Work out the finished part from the listing and answer in its coordinate system (mm). A direction names the side the tool comes from. Coordinates: 2 decimals unless noted, no trailing zeros. Write each loop counter-clockwise with the first axis right and the second up, starting at its lowest first coordinate (ties: lowest second). Pieces come first, ordered by that corner, then holes. Notation, with made-up numbers: (25.5, 84.5) -> (79.5, 84.5) arc R19 ccw to (79.5, 104.5) -> close; hole circle Ø3 at (2.25, 72.25). An arc over 180 degrees is marked (long way). Write each question's results on one line, items separated by ' | '. Start each with the question number.
Autodesk Inventor part; units mm, degrees
ref_plane "Work Plane1" through (-11.4, -3, 12.9) normal (0, 0, -1) x (-1, 0, 0)
ref_plane "Work Plane3" through (-9.3294, -8.5807, 12.9) normal (-0.9659258, 0.258819, 0) x (-0.258819, -0.9659258, 0)
ref_plane "YZ Plane" through (0, 0, 0) normal (1, 0, 0) x (0, 1, 0)
sketch "Sketch1" plane through (0, 0, 0) normal (0, 1, 0) x (-1, 0, 0)
  line L0 (0, 64.7) -> (11.4, 64.7) construction
  line L1 (11.4, 64.7) -> (11.4, 0) construction
  line L2 (11.4, 0) -> (0, 0) construction
  line L3 (0, 0) -> (0, 64.7) construction
  line L4 (5.7, 64.7) -> (5.7, 0) construction
  line L5 (11.4, 32.35) -> (0, 32.35) construction
  circle A0 centre (5.7, 53.1) radius 1.6 construction
  circle A1 centre (5.7, 53.1) radius 2.05
  circle A2 centre (5.7, 43.4) radius 1.6 construction
  circle A3 centre (5.7, 43.4) radius 2.05 construction
  circle A4 centre (5.7, 33.7) radius 1.6 construction
  circle A5 centre (5.7, 33.7) radius 2.05 construction
  circle A6 centre (5.7, 24) radius 1.6 construction
  circle A7 centre (5.7, 24) radius 2.05 construction
  circle A8 centre (5.7, 14.3) radius 1.6 construction
  circle A9 centre (5.7, 14.3) radius 2.05 construction
  circle A10 centre (5.7, 4.6) radius 1.6 construction
  circle A11 centre (5.7, 4.6) radius 2.05
  line L6 (8.2, 64.7) -> (3.2, 64.7) construction
  line L7 (3.2, 64.7) -> (3.2, 0)
  line L8 (3.2, 0) -> (8.2, 0) construction
  line L9 (8.2, 0) -> (8.2, 64.7)
  circle A12 centre (5.7, 53.1) radius 2.5 construction
  circle A13 centre (5.7, 59) radius 5.7 construction
  circle A14 centre (8.2, 3.2) radius 3.2 construction
  line L10 (0, 0) -> (3.2, 0) construction
  line L11 (1.6, 0) -> (1.6, 64.7)
  circle A15 centre (5.7, 4.6) radius 3.65
  circle A16 centre (5.7, 14.3) radius 3.65 construction
  circle A17 centre (5.7, 24) radius 3.65 construction
  circle A18 centre (5.7, 33.7) radius 3.65 construction
  circle A19 centre (5.7, 43.4) radius 3.65 construction
  circle A20 centre (5.7, 53.1) radius 3.65
  arc A21 (8.2, 0) -> (11.4, 3.2) centre (8.2, 3.2) ccw
  arc A22 (11.4, 59) -> (5.7, 64.7) centre (5.7, 59) ccw
  line L12 (11.4, 3.2) -> (11.4, 59)
  line L13 (1.6, 0) -> (8.2, 0)
  line L14 (1.6, 64.7) -> (5.7, 64.7)
  point P0 (5.7, 54.7)
  point P1 (5.7, 3)
  point P2 (-5.6396, 32.0975)
  point P3 (-5.6396, -32.6025)
  point P4 (-1.0396, 31.5935)
  point P5 (8.2, 64.1225)
  point P6 (8.2, 55.7594)
  point P7 (8.2, 50.4406)
  point P8 (3.2, 0)
  point P9 (3.2, 50.4406)
  point P10 (3.2, 55.7594)
  dimension "d4" = 3.2
  dimension "d5" = 4.1
  dimension "d6" = 9.7
  dimension "d7" = 6.5
  dimension "d8" = 10
  dimension "d9" = 3
  dimension "d10" = 0.9
  dimension "d11" = 3.2
  dimension "d12" = 7.3
extrude "Extrusion1" add sketch "Sketch1" along normal blind 6 contours L7 A20 A15 L13 L11 L14 | L7 A20 | A20 L9 | L9 A22 L12 A21 A15 A20 | L7 A15 | A15 L9
extrude "Extrusion2" add sketch "Sketch1" along normal blind 5 contours L14 A22 L9 A20 L7 | A20 L9 L7 | A20 L9 A15 L7 | A15 L9 L7 | L7 A15 L9 L13
extrude "Extrusion3" add sketch "Sketch1" against normal blind 3 contours L14 A22 L9 A20 L7 | L7 A20 A15 L13 L11 L14 | A20 L9 A15 L7 | L9 A22 L12 A21 A15 A20 | L7 A15 L9 L13
sketch "Sketch2" plane through (0, -3, 0) normal (0, -1, 0) x (1, 0, 0)
  line L0 (-5.7, 53.1) -> (-5.7, 4.6) construction
  circle A0 centre (-5.7, 53.1) radius 4.85 construction
  circle A1 centre (-5.7, 43.4) radius 4.85 construction
  circle A2 centre (-5.7, 33.7) radius 4.85 construction
  circle A3 centre (-5.7, 24) radius 4.85 construction
  circle A4 centre (-5.7, 14.3) radius 4.85 construction
  circle A5 centre (-5.7, 4.6) radius 4.85 construction
  line L1 (-11.4, 3.2) -> (-11.4, 59) construction
  line L2 (0, 35.1) -> (-11.4, 35.1) construction
  line L3 (-11.4, 35.1) -> (-11.4, 12.9) construction
  line L4 (-11.4, 12.9) -> (0, 12.9) construction
  line L5 (0, 12.9) -> (0, 35.1) construction
  line L6 (0, 35.1) -> (-11.4, 12.9) construction
  line L7 (-11.4, 35.1) -> (0, 12.9) construction
  point P0 (0, 0)
  dimension "d20" = 22.2
ref_plane "Work Plane1" through (-11.4, -3, 12.9) normal (0, 0, -1) x (-1, 0, 0)
sketch "Sketch3" plane through (-11.4, -3, 12.9) normal (0, 0, -1) x (-1, 0, 0)
  line L0 (0, 0) -> (-9.8, 0)
  line L1 (0, 0) -> (9.8, 0) construction
  line L2 (9.8, 0) -> (9.8, -2.4) construction
  line L3 (0, 0) -> (0, -15.3081)
  line L4 (0, -15.3081) -> (-9.8, -17.934)
  line L5 (-9.8, -17.934) -> (-9.8, 0)
  line L6 (-9.8, -15.934) -> (0, -13.3081)
  line L7 (9.8, -2.4) -> (0, -5.0259) construction
  line L8 (0, -5.0259) -> (-9.8, -7.6518)
  line L9 (9.8, -2.4) -> (0, -2.4) construction
  line L10 (0, -13.3081) -> (-2.0706, -5.5807) construction
  point P0 (-11.4, 3)
  dimension "d32" = 2.4
  dimension "d34" = 15
  dimension "d35" = 8
  dimension "d36" = 2
extrude "Extrusion4" add sketch "Sketch3" along normal blind 2
extrude "Extrusion5" add sketch "Sketch3" against normal blind 22.2 contours L3 L8 L5 L0
extrude "Extrusion6" add sketch "Sketch3" against normal blind 5 contours L3 L4 L5 L6
ref_plane "Work Plane3" through (-9.3294, -8.5807, 12.9) normal (-0.9659258, 0.258819, 0) x (-0.258819, -0.9659258, 0)
sketch "Sketch5" plane through (-9.3294, -8.5807, 12.9) normal (-0.9659258, 0.258819, 0) x (-0.258819, -0.9659258, 0)
  line L0 (0, 0) -> (0, 22.2)
  arc A0 (0, 22.2) -> (0, 0) centre (24.4688, 11.1) ccw
  line L1 (-2.4, 11.1) -> (-2.4, 22.2)
  line L2 (-2.4, 22.2) -> (0, 22.2)
  line L3 (-4.8546, 22.2) -> (0, 22.2)
  point P0 (-10.703, -12.9)
  point P1 (0, 11.1)
  dimension "d37" = 2.4
extrude "Extrusion7" cut sketch "Sketch5" along normal through all both and the other way through all
properties part number "Right-Brush-Top"
1. Find section C-C on x = -5. Give the number of separate pieces and of enclosed holes in the cut face, and give its area (3 significant figures).
2. Find the intervals of material crossed by L1, parallel to Z at x = -5.7, y = 3.65; L2, parallel to Z at x = -5.7, y = -1.15; L3, parallel to X at y = 4.25, z = 53, in increasing order.
3. Find section B-B on z = 32. Give the vertices of the cut face in (x, y).
4. Determine the mould class of faces 6 (the face through (-5, 1, 0)), 7 (the face through (-6, -5, 35.1)), 8 (the face through (-7.3, 0, 51.5)) for opening direction Z: pulls with the +Z half, pulls with the -Z half, needs draft (parallel to the pull), parting line crosses it, or undercut.
5. For faces 1 (the face through (-6.43, -17.64, 15.36)), 2 (the face through (-8, -3, 8)), 3 (the face through (-6.28, -7.56, 18.24)), 4 (the face through (-6.431, -6.873, 29.472)), 5 (the face through (-6, 5, 33)), determine the directions among +Z, -Z, +X, -X, +Y, -Y from which every point of the face is accessible in a straight line to the end or side of a thin tool.
6. Given pin 1 Ø2 at (x, z) = (-5, 42.5) entering from +Y; pin 2 Ø3.5 at (x, z) = (-5.7, 4.6) entering from -Y; pin 3 Ø1.5 at (x, z) = (-2.5, 42) entering from -Y; pin 4 Ø2.5 at (x, y) = (-6, -18.5) entering from +Z, each flat-ended and moving along its own axis, determine where each tip first touches the part or whether it passes through.
7. Find section A-A on z = 53.1. Give the vertices of the cut face in (x, y), and give its area (3 significant figures).
Ans:
1) separate pieces: 3 | enclosed holes: 0 | area: 584 mm²
2) L1: z = 0 to 2.55, 6.65 to 51.05, 55.15 to 64.7 | L2: z = 0 to 0.95, 8.25 to 49.45, 56.75 to 64.7 | L3: x = -11.4 to -7.75, -3.65 to -1.6
3) outline: (-11.4, -5.54) -> (-1.6, -8.17) -> (-1.6, 6) -> (-3.2, 6) -> (-3.2, 5) -> (-8.2, 5) -> (-8.2, 6) -> (-11.4, 6) -> close
4) face 6: pulls with the -Z half | face 7: pulls with the +Z half | face 8: undercut
5) face 1: +Z, +X | face 2: -Z, +X, -X, -Y | face 3: +Z, -X | face 4: +Z, -X, -Y | face 5: +Z, -Z, +Y
6) pin 1: stops at y = 5 | pin 2: passes through | pin 3: stops at y = -3 | pin 4: stops at z = 17.9
7) outline: (-11.4, -3) -> (-9.35, -3) -> (-9.35, 0) -> (-7.75, 0) -> (-7.75, 5) -> (-8.2, 5) -> (-8.2, 6) -> (-11.4, 6) -> close; (-3.65, 0) -> (-2.05, 0) -> (-2.05, -3) -> (-1.6, -3) -> (-1.6, 6) -> (-3.2, 6) -> (-3.2, 5) -> (-3.65, 5) -> close | area: 40.8 mm²
